```python
from build123d import *

# Parameters (mm, degrees)
SKETCH1_R           = 6
BOSS_EXTRUDE1_DEPTH = 12
CHAMFER1_SIZE       = 0.1
CHAMFER1_SIZE2      = 0.123280305
CHAMFER2_SIZE       = 0.5


with BuildPart() as part:
    # Sketch1 → Boss-Extrude1 (new body)
    with BuildSketch(Plane(origin=(0, 0, 0), x_dir=(1, 0, 0), z_dir=(0, 1, 0))):
        with Locations(Location((0, 0, 0), (0, 0, 270))):
            Circle(SKETCH1_R)
    extrude(amount=BOSS_EXTRUDE1_DEPTH)

    # Sketch2 → Cut-Revolve1 (revolve, cut)
    with BuildSketch(Plane.XY, mode=Mode.PRIVATE) as cut_revolve1_sk:
        Polygon((5, 0), (0, 0), (0, 8.5), (1.5, 8.5), (1.5, 4.117144432), (5, 3.5), align=None)
    revolve(cut_revolve1_sk.sketch.rotate(Axis((0, 0, 0), (0, 1, 0)), 90), axis=Axis((0, 0, 0), (0, 1, 0)), mode=Mode.SUBTRACT)

    # Chamfer1
    chamfer1_edges = [part.edges().sort_by_distance(p)[0] for p in [
        (0, 4.117144432, 1.5),
    ]]
    chamfer1_side = [part.faces().sort_by_distance(p)[0] for p in [
        (0, 3.808572216, 3.25),
    ]]
    chamfer(chamfer1_edges, length=CHAMFER1_SIZE, length2=CHAMFER1_SIZE2, reference=chamfer1_side[0])

    # Chamfer2
    chamfer2_edges = [part.edges().sort_by_distance(p)[0] for p in [
        (0, 12, -6),
    ]]
    chamfer(chamfer2_edges, length=CHAMFER2_SIZE)


solid = part.part
```
Design review of the part built by this model. Coordinates are the model's own, in mm. A direction names the side the tool comes from. Coordinates: 2 decimals unless noted, no trailing zeros. Order: outer loops, then holes, each group sorted by start corner. A loop starts at its lowest first (then second) coordinate and runs counter-clockwise, first axis right, second up.
1) Mouldability with a two-part tool opening along X and no side actions: class faces 1 (the flat face through (0, 12, 0)), 2 (the cylindrical face through (1.802, 5.67, 5.723)), 3 (the cylindrical face through (-1.487, 6.34, 0.195)) as +X half, -X half, draft (parallel to the pull), parting line (faces both ways), or undercut.
2) Take a section at A-A, the plane y = 10. Give the boundary of the cut face in (x, z), and give its area (3 significant figures).
3) Clearance check with flat-ended pins moving along their axes: pin 1 (1 mm diameter, centred on x = 3.5, y = 3.5, fed in from -Z); pin 2 (3.5 mm diameter, centred on x = -0.5, z = 0, fed in from -Y); pin 3 (1 mm diameter, centred on x = 2, y = 6.5, fed in from -Z). State where each tip first meets the part, or that it passes through.
4) Take a section at B-B, the plane y = 2.5. Give the boundary of the cut face in (x, z), and give its area (3 significant figures).
5) Wall thickness on line 1 along X through (y, z) = (6.2, 0); line 2 along X through (y, z) = (2.2, 0); line 3 along Z through (x, y) = (-3.5, 2.25): over which ranges is each line inside the solid? List them lowest first.
6) For faces 4 (the flat face through (0, 8.5, 0)), 5 (the flat face through (4, 0, -4)), list the 3-axis set-ups (+Z, -Z, +X, -X, +Y, -Y) from which the entire face can be reached by the end or side of a thin tool; tool diameter is ignored.
Returned:
1. face 1: draft
1. face 2: parting line
1. face 3: undercut
2. outline: circle Ø12 at (0, 0)
2. area: 113 mm2
3. pin 1: stops at z = -5.2
3. pin 2: stops at y = 3.98
3. pin 3: stops at z = -5.81
4. outline: circle Ø12 at (0, 0); hole circle Ø10 at (0, 0)
4. area: 34.6 mm2
5. line 1: x = -6 to -1.5, 1.5 to 6
5. line 2: x = -6 to -5, 5 to 6
5. line 3: z = -4.87 to -3.57, 3.57 to 4.87
6. face 4: -Y
6. face 5: +Z, -Z, +X, -X, -Y
